```python
from build123d import *

# Parameters (mm, degrees)
F2_R = 0.3066051224
F3_R = 0.4318
F4_R = 0.254


# Not quite as in the source:
# - a feature names something its author has since deleted; it is built from what else it names


with BuildPart() as f1:
    # F0 (on Front) → F1 (revolve)
    with BuildSketch(Plane.XZ):
        Polygon((3.9006043464, 21.6174807614), (0.5986043464, 21.6174807614), (0.5986043464, 0), (0.8526043464, 0), (3.3346717246, 3.5295289444), (3.3346717246, 9.5524807614), (2.2496043464, 9.5524807614), (2.2496043464, 11.5844807614), (3.9006043464, 11.5844807614), align=None)
    revolve(axis=Axis((0.5986043464, 0, 10.8087403807), (0, 0, -1)))

    # F2
    f2_edges = [f1.edges().sort_by_distance(p)[0] for p in [
        (-2.703396, 0, 21.617481),
        (-2.703396, 0, 11.584481),
    ]]
    fillet(f2_edges, radius=F2_R)

    # F3
    f3_edges = [f1.edges().sort_by_distance(p)[0] for p in [
        (0.344604, 0, 0),
    ]]
    fillet(f3_edges, radius=F3_R)

    # F4
    f4_edges = [f1.edges().sort_by_distance(p)[0] for p in [
        (-2.137463, 0, 9.552481),
        (-1.052396, 0, 9.552481),
    ]]
    fillet(f4_edges, radius=F4_R)


solid = f1.part
```
Check sheet for the modelled part. Datum: model origin and axes. Units: mm. A direction names the side the tool comes from. Give positions to 0.01 mm unless a question says otherwise; leave off trailing zeros. Write each loop counter-clockwise with the first axis right and the second up, starting at its lowest first coordinate (ties: lowest second). Pieces come first, ordered by that corner, then holes. Notation, with made-up numbers: (7, 54) - (63, 54) arc R25 ccw to (63, 90) - close; hole circle Ø11 at (-9.75, 20). An arc over 180 degrees is marked (long way). Answer as a JSON object with one key per item and string values. Group by question number.
1) Depth check by flat-ended pin: P1, Ø1.5, axis at y = -2.5, z = 11.5, coming from the -X side; P2, Ø3, axis at y = -2, z = 14, coming from the -X side; P3, Ø1, axis at x = 2, z = 2.5, coming from the +Y side. Enter the tip coordinate at first touch or a pass-through.
2) Thickness scan on probe 1 along Y at (x, z) = (0.5, 14.25); probe 2 along Z at (x, y) = (0, -1.75); probe 3 along Z at (x, y) = (-1, -1.5). Record the ranges inside material, lowest first. Write a range as from..to.
3) Sectioned sample at A-A (z = 7). Record the cut outline in (x, y), then the cut area to 3 significant figures.
4) Access from +Z, -Z, +X, -X, +Y, -Y to the whole of each face (thin tool, end or side, straight path). Record for faces 4 (the face through (1, 0, 21.617)), 5 (the face through (0.24, 1.61, 10.71)), 6 (the face through (3.126, 1.048, 6.454)).
5) Release check for a two-part mould opening along Z. For faces 1 (the face through (-0.117, 3.223, 16.667)), 2 (the face through (0, 2, 9.552)), 3 (the face through (0.37, 1.03, 1.14)) record: pulls with the +Z half, pulls with the -Z half, needs draft (parallel to the pull), parting line crosses it, or undercut.
6) Sectioned sample at B-B (z = 18). Record the cut outline in (x, y), then the cut area to 3 significant figures.
Geometry results:
{
 "1": {"P1": "stops at x = -2.15", "P2": "stops at x = -2.67", "P3": "stops at y = 2.01"},
 "2": {"probe 1": "y = -3.3..3.3", "probe 2": "z = 2.27..9.56, 11.58..21.62", "probe 3": "z = 2.76..9.55, 11.58..21.62"},
 "3": {"outline": "circle Ø5.47 at (0.6, 0)", "area": "23.5 mm^2"},
 "4": {"face 4": "+Z, +X, -X, +Y, -Y", "face 5": "none", "face 6": "-Z"},
 "5": {"face 1": "needs draft", "face 2": "undercut", "face 3": "pulls with the -Z half"},
 "6": {"outline": "circle Ø6.6 at (0.6, 0)", "area": "34.3 mm^2"}
}
